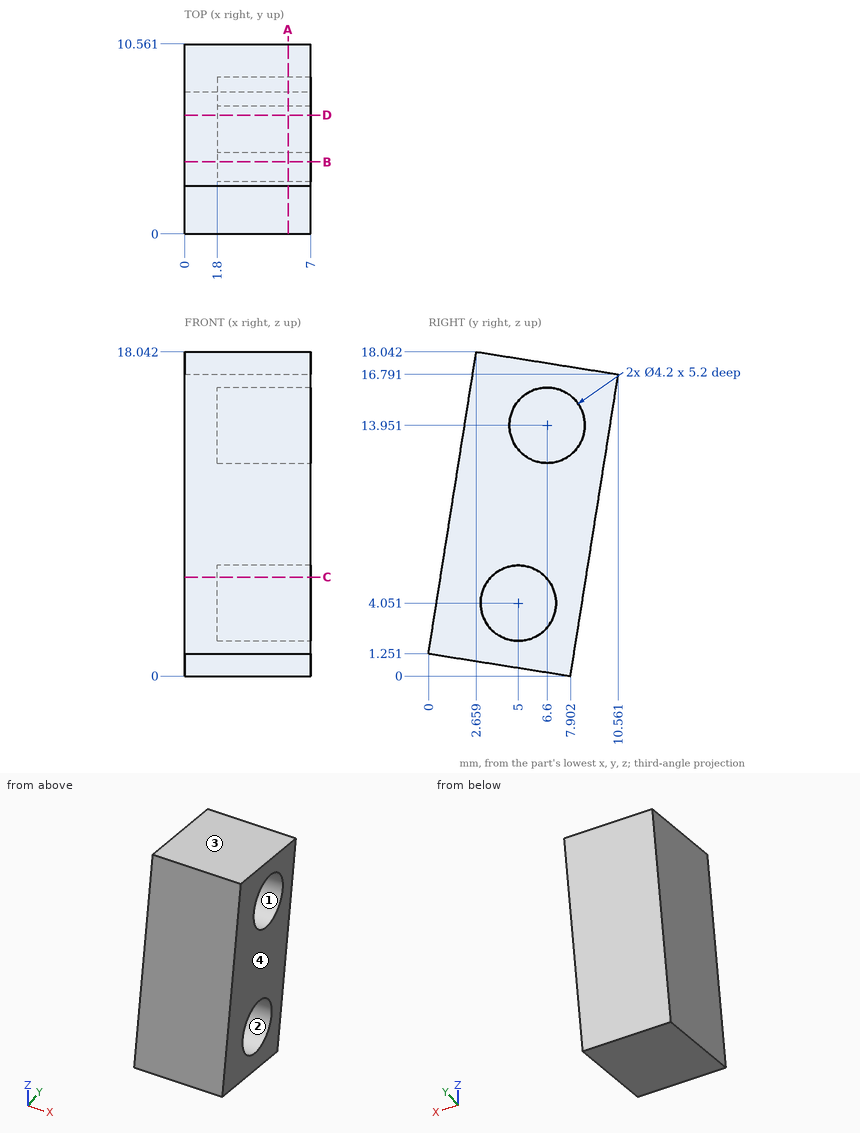
The figure shows three views and two pictorial views of one solid part (mm, origin at its lowest corner). Answer the questions. Coordinates: 2 decimals unless noted, no trailing zeros. Loops run counter-clockwise (first coordinate to the right, second up) from the corner with the lowest first, then second, coordinate; pieces in that order, holes last. Notation, with made-up numbers: (54.25, 88) -> (106.25, 88) arc R17 cw to (106.25, 107) -> close; hole circle Ø9 at (-8.75, 17). An arc over 180 degrees is marked (long way). Write item = value, one per line. Start each with the question number.
1) A cutting plane is placed at D-D (y = 6.6). Give the vertices of the cut face in (x, z).
2) Straight lines are drawn through the part: line 1 (Z direction, x = 4.5, y = 5.5); line 2 (Y direction, x = 5.25, z = 4) (1 decimal); line 3 (Z direction, x = 5, y = 6.25) (1 decimal). For each, find the intervals that lie inside material, in ascending order. Write a range as from..to.
3) A cutting plane is placed at A-A (x = 5.75). Give the vertices of the cut face in (y, z), then the cut area to 3 significant figures.
4) A cutting plane is placed at B-B (y = 4). Give the vertices of the cut face in (x, z) (1 decimal), then the cut area to 3 significant figures.
5) The mould has two halves that part along Y. Classify the marked faces 1, 2, 3 and 4: released by +Y, released by -Y, zero draft, split by the parting line, or undercut.
6) Given pin 1 Ø1 at (y, z) = (4.5, 4.5) entering from -X; pin 2 Ø2 at (y, z) = (7, 14) entering from +X; pin 3 Ø4 at (x, z) = (4.5, 16) entering from -Y; pin 4 Ø1 at (x, z) = (2.5, 3.5) entering from -Y, each flat-ended and moving along its own axis, determine where each tip first touches the part or whether it passes through.
7) A cutting plane is placed at C-C (z = 5.5). Give the vertices of the cut face in (x, y).
Responses:
q1.outline = (0, 0.21) -> (7, 0.21) -> (7, 2.69) -> (1.8, 2.69) -> (1.8, 5.41) -> (7, 5.41) -> (7, 11.85) -> (1.8, 11.85) -> (1.8, 16.05) -> (7, 16.05) -> (7, 17.42) -> (0, 17.42) -> close
q2.line_1 = 0.38..2.01, 6.09..12.16, 15.74..17.59
q2.line_2 = 0.4..2.9, 7.1..8.5
q2.line_3 = 0.3..2.4, 5.7..11.9, 16..17.5
q3.outline = (0, 1.25) -> (7.9, 0) -> (10.56, 16.79) -> (2.66, 18.04) -> close; hole circle Ø4.2 at (5, 4.05); hole circle Ø4.2 at (6.6, 13.95)
q3.area = 108 mm²
q4.outline = (0, 0.6) -> (7, 0.6) -> (7, 2.2) -> (1.8, 2.2) -> (1.8, 5.9) -> (7, 5.9) -> (7, 17.8) -> (0, 17.8) -> close
q4.area = 101 mm²
q5.face_1 = undercut
q5.face_2 = undercut
q5.face_3 = released by +Y
q5.face_4 = zero draft
q6.pin_1 = 0
q6.pin_2 = 1.8
q6.pin_3 = 2.02
q6.pin_4 = 0.28
q7.outline = (0, 0.67) -> (7, 0.67) -> (7, 3.48) -> (1.8, 3.48) -> (1.8, 6.52) -> (7, 6.52) -> (7, 8.77) -> (0, 8.77) -> close
